```python
from build123d import *

# Parameters (mm, degrees)
BOSS_EXTRUDE3_DEPTH   = 6.35
SKETCH13_W            = 12.7
SKETCH13_H            = 6.35
BOSS_EXTRUDE4_DEPTH   = 41.275
SKETCH14_W            = 12.7
SKETCH14_H            = 6.35
SKETCH14_W_2          = 69.85
BOSS_EXTRUDE5_DEPTH   = 6.35
CUT_EXTRUDE4_DEPTH    = 107.917859827
CUT_EXTRUDE5_DEPTH    = 107.917859827
SKETCH26_R            = 2.5
BOSS_EXTRUDE6_DEPTH   = 6.35
BOSS_EXTRUDE7_START   = -47.625
SKETCH26_2_R          = 2.5
BOSS_EXTRUDE7_DEPTH   = 6.35
FILLET17_R            = 1.27
FILLET18_R            = 1.27
FILLET19_R            = 1.27
FILLET20_START        = 47.625
FILLET20_DEPTH        = 6.35
FILLET21_R            = 1.27
FILLET22_DEPTH        = 6.35
FILLET29_R            = 2.54
F_8_CLEARANCE_HOLE1_D = 4.4958
FILLET30_R            = 6.35
FILLET31_R            = 2.54


with BuildPart() as part:
    # Sketch4 → Boss-Extrude3 (new body)
    with BuildSketch(Plane(origin=(0, 0, 0), x_dir=(0, 0, -1), z_dir=(1, 0, 0))):
        Polygon((0, 0), (41.275, 41.275), (82.55, 0), (82.55, -6.35), (0, -6.35), align=None)
    extrude(amount=BOSS_EXTRUDE3_DEPTH)

    # Sketch13 → Boss-Extrude4 (add)
    with BuildSketch(Plane(origin=(6.35, 0, 0), x_dir=(0, 0, -1), z_dir=(1, 0, 0))):
        with Locations((6.35, -3.175)):
            Rectangle(SKETCH13_W, SKETCH13_H)
        with Locations((76.2, -3.175)):
            Rectangle(SKETCH13_W, SKETCH13_H)
    extrude(amount=BOSS_EXTRUDE4_DEPTH)

    # Sketch14 → Boss-Extrude5 (add)
    with BuildSketch(Plane(origin=(47.625, 0, 0), x_dir=(0, 0, -1), z_dir=(1, 0, 0))):
        Polygon((41.275, 41.275), (0, 0), (12.7, 0), (82.55, 0), align=None)
        with Locations((6.35, -3.175)):
            Rectangle(SKETCH14_W, SKETCH14_H)
        with Locations((47.625, -3.175)):
            Rectangle(SKETCH14_W_2, SKETCH14_H)
    extrude(amount=BOSS_EXTRUDE5_DEPTH)

    # Sketch20 → Cut-Extrude4 (cut, through all)
    with BuildSketch(Plane(origin=(53.975, 0, 0), x_dir=(0, 0, -1), z_dir=(1, 0, 0))):
        Polygon((41.275, 28.575), (12.7, 0), (69.85, 0), align=None)
    extrude(amount=-CUT_EXTRUDE4_DEPTH, mode=Mode.SUBTRACT)

    # Sketch21 → Cut-Extrude5 (cut, through all)
    with BuildSketch(Plane(origin=(53.975, 0, 0), x_dir=(0, 0, -1), z_dir=(1, 0, 0))):
        with BuildLine():
            ThreePointArc((43.775, 34.925), (43.042766953, 36.692766953), (41.275, 37.425))
            Line((41.275, 37.425), (41.275, 32.425))
            ThreePointArc((41.275, 32.425), (43.042766953, 33.157233047), (43.775, 34.925))
        make_face()
        with BuildLine():
            Line((41.275, 32.425), (41.275, 37.425))
            ThreePointArc((41.275, 37.425), (38.775, 34.925), (41.275, 32.425))
        make_face()
    extrude(amount=-CUT_EXTRUDE5_DEPTH, mode=Mode.SUBTRACT)

    # Sketch26 → Boss-Extrude6 (add)
    with BuildSketch(Plane.ZY):
        Polygon((-41.275, 41.275), (-80.659092999, 45.187499922), (-133.595070682, 45.187499922), (-88.943397116, -6.35), (-77.720070682, -6.35), (-77.720070682, 35.323646113), (-49.981920931, 32.568079069), align=None)
        with Locations((-80.895070682, 40.424999922)):
            Circle(SKETCH26_R, mode=Mode.SUBTRACT)
        with Locations((-120.895070682, 40.424999922)):
            Circle(SKETCH26_R, mode=Mode.SUBTRACT)
        Polygon((-87.245070682, 35.662499922), (-87.245070682, 6.23593212), (-112.740011292, 35.662499922), align=None, mode=Mode.SUBTRACT)
    extrude(amount=-BOSS_EXTRUDE6_DEPTH)

    # Sketch26<2> → Boss-Extrude7 (add)
    with BuildSketch(Plane.ZY.offset(BOSS_EXTRUDE7_START)):
        Polygon((-41.275, 41.275), (-80.659092999, 45.187499922), (-133.595070682, 45.187499922), (-88.943397116, -6.35), (-77.720070682, -6.35), (-77.720070682, 35.323646113), (-49.981920931, 32.568079069), align=None)
        with Locations((-80.895070682, 40.424999922)):
            Circle(SKETCH26_2_R, mode=Mode.SUBTRACT)
        with Locations((-120.895070682, 40.424999922)):
            Circle(SKETCH26_2_R, mode=Mode.SUBTRACT)
        Polygon((-87.245070682, 35.662499922), (-87.245070682, 6.23593212), (-112.740011292, 35.662499922), align=None, mode=Mode.SUBTRACT)
    extrude(amount=-BOSS_EXTRUDE7_DEPTH)

    # Fillet17
    fillet17_edges = [part.edges().sort_by_distance(p)[0] for p in [
        (3.175, 28.575, -41.275),
    ]]
    fillet(fillet17_edges, radius=FILLET17_R)

    # Fillet18
    fillet18_edges = [part.edges().sort_by_distance(p)[0] for p in [
        (50.8, 28.575, -41.275),
    ]]
    fillet(fillet18_edges, radius=FILLET18_R)

    # Fillet19
    # the kernel refuses this fillet: 1.27 mm, written as the material it adds along each edge
    with BuildSketch(Plane(origin=(53.975, 0, -12.7), x_dir=(0, 0.7071067811865481, -0.7071067811865469), z_dir=(-1, 0, 0))) as fillet19_piece_1:
        with BuildLine():
            CenterArc((FILLET19_R * 2.41421356237, FILLET19_R), FILLET19_R, 135, 135)
            Line((FILLET19_R * 1.70710678119, FILLET19_R * 1.70710678119), (0, 0))
            Line((0, 0), (FILLET19_R * 2.41421356237, 0))
        make_face()
    extrude(amount=6.35)

    # Fillet20: read off the stored shape, not the designer's step
    # Fillet20 outline → Fillet20 (add)
    with BuildSketch(Plane.YZ.offset(FILLET20_START)):
        with BuildLine():
            Line((0, -69.85), (2.168025612, -67.681974388))
            ThreePointArc((2.168025612, -67.681974388), (0.783992041, -67.957275782), (0, -66.783948776))
            Line((0, -66.783948776), (0, -69.85))
        make_face()
    extrude(amount=FILLET20_DEPTH)

    # Fillet21
    # the kernel refuses this fillet: 1.27 mm, written as the material it adds along each edge
    with BuildSketch(Plane(origin=(6.35, 0, -69.85), x_dir=(0, 0, 1), z_dir=(-1, 0, 0))) as fillet21_piece_1:
        with BuildLine():
            CenterArc((FILLET21_R * 2.41421356237, FILLET21_R), FILLET21_R, 135, 135)
            Line((FILLET21_R * 1.70710678119, FILLET21_R * 1.70710678119), (0, 0))
            Line((0, 0), (FILLET21_R * 2.41421356237, 0))
        make_face()
    extrude(amount=6.35)

    # Fillet22: read off the stored shape, not the designer's step
    # Fillet22 outline → Fillet22 (add)
    with BuildSketch(Plane.YZ):
        with BuildLine():
            ThreePointArc((0, -15.766051224), (0.783992041, -14.592724218), (2.168025612, -14.868025612))
            Line((2.168025612, -14.868025612), (0, -12.7))
            Line((0, -12.7), (0, -15.766051224))
        make_face()
    extrude(amount=FILLET22_DEPTH)

    # Fillet29
    fillet29_edges = [part.edges().sort_by_distance(p)[0] for p in [
        (26.9875, 0, -12.7),
        (26.9875, 0, -69.85),
    ]]
    fillet(fillet29_edges, radius=FILLET29_R)

    # #8 Clearance Hole1 (through all)
    with Locations(Plane(origin=(0, 0, 0), x_dir=(1, 0, 0), z_dir=(0, 1, 0))):
        with Locations((16.51, 77.47), (37.465, 77.47), (37.465, 5.08), (16.51, 5.08)):
            Hole(F_8_CLEARANCE_HOLE1_D / 2)

    # Fillet30
    # the kernel refuses this fillet: 6.35 mm, written as the material it takes off along each edge
    with BuildSketch(Plane(origin=(-0.786592277, 45.187499922, -80.659092999), x_dir=(0, -0.0988555378398254, 0.995101795113645), z_dir=(1, 0, 0))) as fillet30_piece_1:
        with BuildLine():
            CenterArc((FILLET30_R * 0.0495491197902, FILLET30_R), FILLET30_R, 264.326728924, 5.673271076)
            Line((-FILLET30_R * 0.0493064180496, FILLET30_R * 0.00489820488635), (0, 0))
            Line((0, 0), (FILLET30_R * 0.0495491197903, 0))
        make_face()
    extrude(amount=7.923184553, mode=Mode.SUBTRACT)
    with BuildSketch(Plane(origin=(46.838407723, 45.187499922, -80.659092999), x_dir=(0, 0, -1), z_dir=(1, 0, 0))) as fillet30_piece_2:
        with BuildLine():
            CenterArc((FILLET30_R * 0.0495491197903, -FILLET30_R), FILLET30_R, 90, 5.673271076)
            Line((-FILLET30_R * 0.0493064180496, -FILLET30_R * 0.00489820488636), (0, 0))
            Line((0, 0), (FILLET30_R * 0.0495491197903, 0))
        make_face()
    extrude(amount=7.923184553, mode=Mode.SUBTRACT)
    with BuildSketch(Plane(origin=(41.952376432, 41.275, -41.275), x_dir=(0, -0.7071067811865476, 0.7071067811865476), z_dir=(1, 0, 0)), Plane(origin=(-5.672623568, 41.275, -41.275), x_dir=(0, -0.7071067811865459, 0.707106781186549), z_dir=(1, 0, 0))) as fillet30_piece_3:
        with BuildLine():
            CenterArc((FILLET30_R * 0.357330618477, FILLET30_R), FILLET30_R, 230.673271076, 39.326728924)
            Line((-FILLET30_R * 0.276411187654, FILLET30_R * 0.22645535154), (0, 0))
            Line((0, 0), (FILLET30_R * 0.357330618477, 0))
        make_face()
    extrude(amount=17.695247137, mode=Mode.SUBTRACT)

    # Fillet31
    fillet31_edges = [part.edges().sort_by_distance(p)[0] for p in [
        (3.175, 35.323646113, -77.720070682),
        (3.175, 32.568079069, -49.981920931),
        (3.175, 4.829929318, -77.720070682),
        (3.175, 45.187499922, -133.595070682),
        (3.175, 35.662499922, -87.245070682),
        (3.175, 6.23593212, -87.245070682),
        (3.175, 35.662499922, -112.740011292),
        (50.8, 4.829929318, -77.720070682),
        (50.8, 35.323646113, -77.720070682),
        (50.8, 32.568079069, -49.981920931),
        (50.8, 45.187499922, -133.595070682),
        (50.8, 35.662499922, -87.245070682),
        (50.8, 35.662499922, -112.740011292),
        (50.8, 6.23593212, -87.245070682),
    ]]
    fillet(fillet31_edges, radius=FILLET31_R)


solid = part.part
```
The model under review builds one solid part; all positions refer to its coordinate system, in mm. A direction names the side the tool comes from. Coordinates: 2 decimals unless noted, no trailing zeros. Write each loop counter-clockwise with the first axis right and the second up, starting at its lowest first coordinate (ties: lowest second). Pieces come first, ordered by that corner, then holes.
1) The part is to be moulded in two halves that separate along Z. For faces 6 (the face through (3.131, 17.648, -109.735)), 7 (the face through (3.2, 15.1, -27.8)), 8 (the face through (51, 20, -20)), say which applies: pulls with the +Z half, pulls with the -Z half, needs draft (parallel to the pull), parting line crosses it, or undercut.
2) We need section A-A on x = 16.51. State the section outline as (y, z) points.
3) We need section D-D on y = 5. State the section outline as (x, z) points (3 decimals), then the cut area to 3 significant figures.
4) We need section C-C on x = 31. State the section outline as (y, z) points.
5) To check wall thickness, follow probe 1 along Y at (x, z) = (2, -60.5); probe 2 along X at (y, z) = (4, -9) (3 decimals); probe 3 along Z at (x, y) = (16, -2). State the ranges of each line that lie inside material, in increasing order.
6) We need section B-B on z = -5.08. State the section outline as (x, y) points (3 decimals), then the cut area to 3 significant figures.
7) Clearance check with flat-ended pins moving along their axes: pin 1 Ø11 at (x, z) = (24, -5) entering from +Y; pin 2 Ø7 at (x, y) = (50.5, 24.5) entering from +Z; pin 3 Ø5 at (x, z) = (4, -99.5) entering from -Y. State where each tip first meets the part, or that it passes through.
8) Machinability: for faces 1 (the face through (39.249, -3.219, -3.712)), 2 (the face through (50.756, 17.648, -109.735)), 3 (the face through (50.756, 34.086, -65.262)), 4 (the face through (27.276, -0.764, -11.976)), 5 (the face through (27, -3, -82.55)), which of the approach directions +Z, -Z, +X, -X, +Y, -Y give a long, thin tool a straight path to every point of the face, cutting with its end or side? Answer none if there is none.
Answer list:
1. face 6: pulls with the -Z half
1. face 7: undercut
1. face 8: pulls with the +Z half
2. outline: (-6.35, -82.55) - (0, -82.55) - (0, -79.72) - (-6.35, -79.72) - close; (-6.35, -75.22) - (0, -75.22) - (0, -72.39) arc R2.54 ccw to (-2.54, -69.85) - (-6.35, -69.85) - close; (-6.35, -12.7) - (-2.54, -12.7) arc R2.54 ccw to (0, -10.16) - (0, -7.33) - (-6.35, -7.33) - close; (-6.35, -2.83) - (0, -2.83) - (0, 0) - (-6.35, 0) - close
3. outline: (0, -98.777) - (6.35, -98.777) - (6.35, -64.85) - (0, -64.85) - close; (0, -17.7) - (6.35, -17.7) - (6.35, -5) - (0, -5) - close; (47.625, -98.777) - (53.975, -98.777) - (53.975, -64.85) - (47.625, -64.85) - close; (47.625, -17.7) - (53.975, -17.7) - (53.975, -5) - (47.625, -5) - close
3. area: 592 mm2
4. outline: (-6.35, -82.55) - (0, -82.55) - (0, -72.39) arc R2.54 ccw to (-2.54, -69.85) - (-6.35, -69.85) - close; (-6.35, -12.7) - (-2.54, -12.7) arc R2.54 ccw to (0, -10.16) - (0, 0) - (-6.35, 0) - close
5. probe 1: y = -6.35 to 0, 9.35 to 22.05, 33.61 to 43.18
5. probe 2: x = 0 to 6.35, 47.625 to 53.975
5. probe 3: z = -82.55 to -79.66, -75.28 to -69.91, -12.64 to -7.27, -2.89 to 0
6. outline: (0, -6.35) - (14.262, -6.35) - (14.262, 0) - (6.35, 0) - (6.35, 5.08) - (0, 5.08) - close; (18.758, -6.35) - (35.217, -6.35) - (35.217, 0) - (18.758, 0) - close; (39.713, -6.35) - (53.975, -6.35) - (53.975, 5.08) - (47.625, 5.08) - (47.625, 0) - (39.713, 0) - close
6. area: 350 mm2
7. pin 1: stops at y = 0
7. pin 2: stops at z = -21
7. pin 3: stops at y = 2.95
8. face 1: +Y, -Y
8. face 2: -Z, +X, -X, -Y
8. face 3: +X, -X
8. face 4: +Y
8. face 5: -Z, +Y, -Y
